Autodesk Inventor part; units mm, degrees
ref_plane "YZ Plane" through (0, 0, 0) normal (1, 0, 0) x (0, 1, 0)
ref_plane "XY Plane" through (0, 0, 0) normal (0, 0, 1) x (1, 0, 0)
sketch "Sketch1" plane through (0, 0, 0) normal (1, 0, 0) x (0, 1, 0)
  circle A0 centre (0, 0) radius 69.85
  circle A1 centre (0, 0) radius 76.2
  dimension "d0" = 139.7
  dimension "d1" = 152.4
extrude "Extrusion1" add sketch "Sketch1" along normal blind 76.2
sketch "Sketch2" plane through (0, 0, 0) normal (0, 1, 0) x (-1, 0, 0)
  line L0 (-76.2, 76.2) -> (-76.2, -76.2)
  line L1 (0, -76.2) -> (-76.2, -76.2)
  line L2 (-76.2, 76.2) -> (-54.61, 76.2)
  line L3 (-54.61, 76.2) -> (-54.61, -76.2)
  line L4 (-54.61, -76.2) -> (-76.2, -76.2)
  line L5 (-76.2, -76.2) -> (-76.2, 76.2)
  point P0 (0, 0)
  dimension "d4" = 21.59
extrude "Extrusion2" cut sketch "Sketch2" against normal blind 76.2
properties part number "hopper v1"
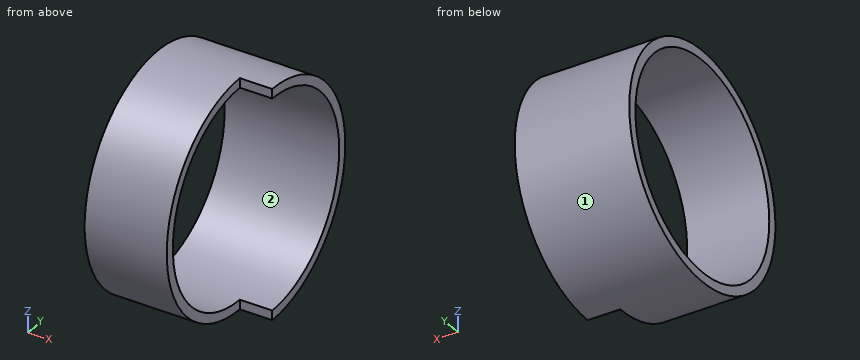
Check sheet for the modelled part. Datum: model origin and axes. Units: mm. Face numbers are marked on the shaded views. Coordinates: 2 decimals unless noted, no trailing zeros. Order: outer loops, then holes, each group sorted by start corner. A loop starts at its lowest first (then second) coordinate and runs counter-clockwise, first axis right, second up. Notation, with made-up numbers: (-30, -5.75) -> (22, -5.75) arc R16 cw to (22, 5.25) -> close; hole circle Ø7 at (-1.75, -37). An arc over 180 degrees is marked (long way). Write item = value, one per line. Start each with the question number.
1) Cross-section at C-C (x = 14). Enter the section's corners in (y, z).
2) Material ranges on L1, parallel to Y at x = 23, z = 0; L2, parallel to Z at x = 17, y = -21, recorded low to high.
3) Cross-section at A-A (z = 0). Enter the section's corners in (x, y).
4) Mould release check, pull along Y, two halves, no side actions. Record for the marked faces 1 and 2: +Y half, -Y half, draft (parallel to the pull), parting line (faces both ways), or undercut.
5) Go/stop test with flat-tipped pins: P1, Ø1.9, axis at x = 70, z = 72.5, coming from the -Y side; P2, Ø3, axis at x = 20, z = 41, coming from the -Y side; P3, Ø5, axis at x = 41, z = 37, coming from the -Y side. Record where each tip stops, or that it passes through.
6) Cross-section at B-B (y = -36). Enter the section's corners in (x, z), then the cut area to 3 significant figures.
Ans:
q1.outline = circle Ø152.4 at (0, 0); hole circle Ø139.7 at (0, 0)
q2.L1 = -76.2 to -69.85, 69.85 to 76.2
q2.L2 = -73.25 to -66.62, 66.62 to 73.25
q3.outline = (0, -76.2) -> (54.61, -76.2) -> (54.61, -69.85) -> (0, -69.85) -> close; (0, 69.85) -> (76.2, 69.85) -> (76.2, 76.2) -> (0, 76.2) -> close
q4.face_1 = parting line
q4.face_2 = undercut
q5.P1 = 0
q5.P2 = -65.16
q5.P3 = -67.94
q6.outline = (0, -67.16) -> (54.61, -67.16) -> (54.61, -59.86) -> (0, -59.86) -> close; (0, 59.86) -> (54.61, 59.86) -> (54.61, 67.16) -> (0, 67.16) -> close
q6.area = 797 mm²
